Design review of the part built by this model. Coordinates are the model's own, in mm. Coordinates: 2 decimals unless noted, no trailing zeros. Write each loop counter-clockwise with the first axis right and the second up, starting at its lowest first coordinate (ties: lowest second). Pieces come first, ordered by that corner, then holes. Notation, with made-up numbers: M 57,-10.75 L 103,-10.75 A9 cw 103,5.25 Z; hole C 13,28 d2. An arc over 180 degrees is marked long. Write item = value, one per line.
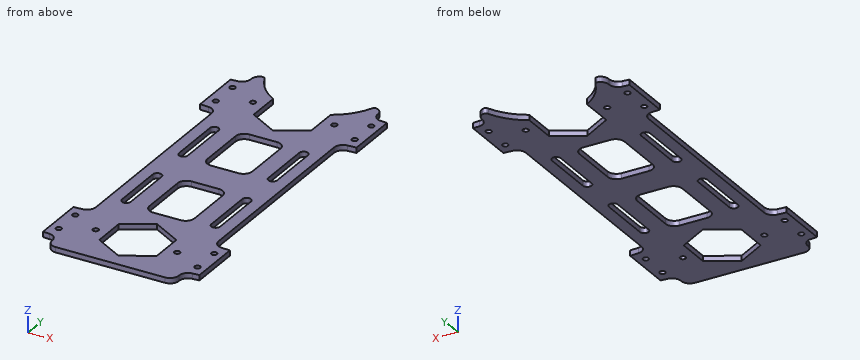
```python
from build123d import *

# Parameters (mm, degrees)
F0_R     = 1.6
F1_DEPTH = 3
F3_DEPTH = 25
F4_R     = 2


with BuildPart() as f1:
    # F0 (on Top) → F1 (new body)
    with BuildSketch(Plane.XY):
        with BuildLine():
            Line((-44.408627, -61.525488), (-44.408627, -91.060406))
            Line((-44.408627, -91.060406), (-40.651218, -91.32315))
            ThreePointArc((-40.651218, -91.32315), (-37.343231, -92.900978), (-36, -96.31097))
            Line((-36, -96.31097), (-36, -96.648395))
            ThreePointArc((-36, -96.648395), (-34.535534, -100.183929), (-31, -101.648395))
            Line((-31, -101.648395), (0, -101.648395))
            Line((0, -101.648395), (31, -101.648395))
            ThreePointArc((31, -101.648395), (34.535534, -100.183929), (36, -96.648395))
            Line((36, -96.648395), (36, -96.31097))
            ThreePointArc((36, -96.31097), (37.343231, -92.900978), (40.651218, -91.32315))
            Line((40.651218, -91.32315), (44.408627, -91.060406))
            Line((44.408627, -91.060406), (44.408627, -61.525488))
            Line((44.408627, -61.525488), (39.450638, -61.178791))
            ThreePointArc((39.450638, -61.178791), (36.142652, -59.600963), (34.799421, -56.190971))
            Line((34.799421, -56.190971), (34.799421, 0))
            Line((34.799421, 0), (34.799421, 56.190971))
            ThreePointArc((34.799421, 56.190971), (36.142652, 59.600963), (39.450638, 61.178791))
            Line((39.450638, 61.178791), (44.408627, 61.525488))
            Line((44.408627, 61.525488), (44.408627, 91.060406))
            Line((44.408627, 91.060406), (40.651218, 91.32315))
            ThreePointArc((40.651218, 91.32315), (37.343231, 92.900978), (36, 96.31097))
            Line((36, 96.31097), (36, 96.648395))
            ThreePointArc((36, 96.648395), (34.535534, 100.183929), (31, 101.648395))
            Line((31, 101.648395), (-31, 101.648395))
            ThreePointArc((-31, 101.648395), (-34.535534, 100.183929), (-36, 96.648395))
            Line((-36, 96.648395), (-36, 96.31097))
            ThreePointArc((-36, 96.31097), (-37.343231, 92.900978), (-40.651218, 91.32315))
            Line((-40.651218, 91.32315), (-44.408627, 91.060406))
            Line((-44.408627, 91.060406), (-44.408627, 61.525488))
            Line((-44.408627, 61.525488), (-39.450638, 61.178791))
            ThreePointArc((-39.450638, 61.178791), (-36.142652, 59.600963), (-34.799421, 56.190971))
            Line((-34.799421, 56.190971), (-34.799421, 0))
            Line((-34.799421, 0), (-34.799421, -56.190971))
            ThreePointArc((-34.799421, -56.190971), (-36.142652, -59.600963), (-39.450638, -61.178791))
            Line((-39.450638, -61.178791), (-44.408627, -61.525488))
        make_face()
        with Locations((-39.408627, -84.392947)):
            Circle(F0_R, mode=Mode.SUBTRACT)
        with Locations((-23.110468, -76.292947)):
            Circle(F0_R, mode=Mode.SUBTRACT)
        with Locations((-39.408627, -68.192947)):
            Circle(F0_R, mode=Mode.SUBTRACT)
        with BuildLine():
            ThreePointArc((-22.877386, -42.681136), (-23.609619, -44.448903), (-25.377386, -45.181136))
            ThreePointArc((-25.377386, -45.181136), (-27.145153, -44.448903), (-27.877386, -42.681136))
            Line((-27.877386, -42.681136), (-27.877386, -12.681136))
            ThreePointArc((-27.877386, -12.681136), (-27.145153, -10.913369), (-25.377386, -10.181136))
            ThreePointArc((-25.377386, -10.181136), (-23.609619, -10.913369), (-22.877386, -12.681136))
            Line((-22.877386, -12.681136), (-22.877386, -42.681136))
        make_face(mode=Mode.SUBTRACT)
        Polygon((16.318487, -65.480797), (16.364526, -84.350343), (0.046039, -93.824987), (-16.318487, -84.430085), (-16.364526, -65.560539), (-0.046039, -56.085895), align=None, mode=Mode.SUBTRACT)
        with Locations((23.110468, -76.292947)):
            Circle(F0_R, mode=Mode.SUBTRACT)
        with Locations((39.408627, -84.392947)):
            Circle(F0_R, mode=Mode.SUBTRACT)
        with Locations((39.408627, -68.192947)):
            Circle(F0_R, mode=Mode.SUBTRACT)
        with BuildLine():
            ThreePointArc((12.763027, -41.744589), (11.298561, -45.280123), (7.763027, -46.744589))
            Line((7.763027, -46.744589), (-7.763027, -46.744589))
            ThreePointArc((-7.763027, -46.744589), (-11.298561, -45.280123), (-12.763027, -41.744589))
            Line((-12.763027, -41.744589), (-12.763027, -14.446382))
            ThreePointArc((-12.763027, -14.446382), (-11.298561, -10.910848), (-7.763027, -9.446382))
            Line((-7.763027, -9.446382), (7.763027, -9.446382))
            ThreePointArc((7.763027, -9.446382), (11.298561, -10.910848), (12.763027, -14.446382))
            Line((12.763027, -14.446382), (12.763027, -41.744589))
        make_face(mode=Mode.SUBTRACT)
        with BuildLine():
            ThreePointArc((25.377386, -45.181136), (23.609619, -44.448903), (22.877386, -42.681136))
            Line((22.877386, -42.681136), (22.877386, -12.681136))
            ThreePointArc((22.877386, -12.681136), (23.609619, -10.913369), (25.377386, -10.181136))
            ThreePointArc((25.377386, -10.181136), (27.145153, -10.913369), (27.877386, -12.681136))
            Line((27.877386, -12.681136), (27.877386, -42.681136))
            ThreePointArc((27.877386, -42.681136), (27.145153, -44.448903), (25.377386, -45.181136))
        make_face(mode=Mode.SUBTRACT)
        with BuildLine():
            ThreePointArc((-22.877386, 12.681136), (-23.609619, 10.913369), (-25.377386, 10.181136))
            ThreePointArc((-25.377386, 10.181136), (-27.145153, 10.913369), (-27.877386, 12.681136))
            Line((-27.877386, 12.681136), (-27.877386, 42.681136))
            ThreePointArc((-27.877386, 42.681136), (-27.145153, 44.448903), (-25.377386, 45.181136))
            ThreePointArc((-25.377386, 45.181136), (-23.609619, 44.448903), (-22.877386, 42.681136))
            Line((-22.877386, 42.681136), (-22.877386, 12.681136))
        make_face(mode=Mode.SUBTRACT)
        with Locations((-39.408627, 68.192947)):
            Circle(F0_R, mode=Mode.SUBTRACT)
        with Locations((-39.408627, 84.392947)):
            Circle(F0_R, mode=Mode.SUBTRACT)
        with Locations((-23.110468, 76.292947)):
            Circle(F0_R, mode=Mode.SUBTRACT)
        with BuildLine():
            ThreePointArc((12.763027, 14.446382), (11.298561, 10.910848), (7.763027, 9.446382))
            Line((7.763027, 9.446382), (-7.763027, 9.446382))
            ThreePointArc((-7.763027, 9.446382), (-11.298561, 10.910848), (-12.763027, 14.446382))
            Line((-12.763027, 14.446382), (-12.763027, 41.744589))
            ThreePointArc((-12.763027, 41.744589), (-11.298561, 45.280123), (-7.763027, 46.744589))
            Line((-7.763027, 46.744589), (7.763027, 46.744589))
            ThreePointArc((7.763027, 46.744589), (11.298561, 45.280123), (12.763027, 41.744589))
            Line((12.763027, 41.744589), (12.763027, 14.446382))
        make_face(mode=Mode.SUBTRACT)
        with BuildLine():
            ThreePointArc((22.877386, 42.681136), (23.609619, 44.448903), (25.377386, 45.181136))
            ThreePointArc((25.377386, 45.181136), (27.145153, 44.448903), (27.877386, 42.681136))
            Line((27.877386, 42.681136), (27.877386, 12.681136))
            ThreePointArc((27.877386, 12.681136), (27.145153, 10.913369), (25.377386, 10.181136))
            ThreePointArc((25.377386, 10.181136), (23.609619, 10.913369), (22.877386, 12.681136))
            Line((22.877386, 12.681136), (22.877386, 42.681136))
        make_face(mode=Mode.SUBTRACT)
        Polygon((-0.046039, 56.085895), (-16.364526, 65.560539), (-16.318487, 84.430085), (0.046039, 93.824987), (16.364526, 84.350343), (16.318487, 65.480797), align=None, mode=Mode.SUBTRACT)
        with Locations((39.408627, 68.192947)):
            Circle(F0_R, mode=Mode.SUBTRACT)
        with Locations((23.110468, 76.292947)):
            Circle(F0_R, mode=Mode.SUBTRACT)
        with Locations((39.408627, 84.392947)):
            Circle(F0_R, mode=Mode.SUBTRACT)
    extrude(amount=F1_DEPTH)

    # F2 (on Top) → F3 (cut)
    with BuildSketch(Plane.XY):
        with BuildLine():
            Line((31, 101.648395), (-31, 101.648395))
            ThreePointArc((-31, 101.648395), (-11.329383, 82.014911), (16.364526, 84.350343))
            ThreePointArc((16.364526, 84.350343), (25.212204, 91.704922), (31, 101.648395))
        make_face()
    extrude(amount=F3_DEPTH, mode=Mode.SUBTRACT)

    # F4
    f4_edges = [f1.edges().sort_by_distance(p)[0] for p in [
        (31, 101.648395, 1.5),
        (-31, 101.648395, 1.5),
    ]]
    fillet(f4_edges, radius=F4_R)


solid = f1.part
```
Q1. For P1, Ø1.5, axis at y = 23.5, z = 1.5, coming from the +X side; P2, Ø1.5, axis at y = -23, z = 2, coming from the -X side; P3, Ø1.5, axis at x = -2.5, z = 2, coming from the +Y side, all flat-tipped, find the tip position at first contact; note any pin that passes through.
Check result:
P1 = 34.8
P2 = -34.8
P3 = 57.95
Q2. Consider section C-C, the plane z = 2.3. State how many separate pieces and enclosed holes the cut face has, and give its area (3 significant figures).
Check result:
separate_pieces = 1
enclosed_holes = 19
area = 10,200 mm²
Q3. Consider section B-B, the plane y = 58. State the section outline as (x, z) points.
Check result:
outline = M -35.14,0 L -3.34,0 L -3.34,3 L -35.14,3 Z; M 3.29,0 L 35.14,0 L 35.14,3 L 3.29,3 Z
Q4. Consider section A-A, the plane y = 36.5. State the section outline as (x, z) points.
Check result:
outline = M -34.8,0 L -27.88,0 L -27.88,3 L -34.8,3 Z; M -22.88,0 L -12.76,0 L -12.76,3 L -22.88,3 Z; M 12.76,0 L 22.88,0 L 22.88,3 L 12.76,3 Z; M 27.88,0 L 34.8,0 L 34.8,3 L 27.88,3 Z
Q5. Wall thickness on line 1 (X direction, y = -25, z = 1.9); line 2 (Y direction, x = -4.5, z = 2.45); line 3 (X direction, y = -78.5, z = 0.6): over which ranges is each line inside the solid? List them lowest first.
Check result:
line_1 = -34.8 to -27.88, -22.88 to -12.76, 12.76 to 22.88, 27.88 to 34.8
line_2 = -101.65 to -91.22, -58.67 to -46.74, -9.45 to 9.45, 46.74 to 58.67
line_3 = -44.41 to -16.33, 16.35 to 44.41
